```python
from build123d import *

# Parameters (mm, degrees)
SKETCH1_R           = 7
BOSS_EXTRUDE1_DEPTH = 2
SKETCH2_R           = 5.95
BOSS_EXTRUDE2_DEPTH = 7
SKETCH3_W           = 3.8
SKETCH3_H           = 3.8
CUT_EXTRUDE1_DEPTH  = 1.8
CHAMFER1_SIZE       = 1


with BuildPart() as part:
    # Sketch1 → Boss-Extrude1 (new body)
    with BuildSketch(Plane(origin=(0, 0, 0), x_dir=(1, 0, 0), z_dir=(0, 1, 0))):
        with Locations(Location((0, 0, 0), (0, 0, 270))):
            Circle(SKETCH1_R)
    extrude(amount=BOSS_EXTRUDE1_DEPTH)

    # Sketch2 → Boss-Extrude2 (add)
    with BuildSketch(Plane(origin=(0, 2, 0), x_dir=(1, 0, 0), z_dir=(0, 1, 0))):
        with Locations(Location((0, 0, 0), (0, 0, 270))):
            Circle(SKETCH2_R)
    extrude(amount=BOSS_EXTRUDE2_DEPTH)

    # Sketch3 → Cut-Extrude1 (cut)
    with BuildSketch(Plane.XZ):
        with BuildLine():
            ThreePointArc((-1.9, 1.9), (-2.687005769, 0), (-1.9, -1.9))
            Line((-1.9, -1.9), (-1.9, 1.9))
        make_face()
        Rectangle(SKETCH3_W, SKETCH3_H)
        with BuildLine():
            ThreePointArc((1.9, 1.9), (0, 2.687005769), (-1.9, 1.9))
            Line((-1.9, 1.9), (1.9, 1.9))
        make_face()
        with BuildLine():
            Line((1.9, 1.9), (1.9, -1.9))
            ThreePointArc((1.9, -1.9), (2.482469633, -1.02827259), (2.687005769, 0))
            ThreePointArc((2.687005769, 0), (2.482469633, 1.02827259), (1.9, 1.9))
        make_face()
        with BuildLine():
            Line((1.9, -1.9), (-1.9, -1.9))
            ThreePointArc((-1.9, -1.9), (0, -2.687005769), (1.9, -1.9))
        make_face()
    extrude(amount=-CUT_EXTRUDE1_DEPTH, mode=Mode.SUBTRACT)

    # Chamfer1
    chamfer1_edges = [part.edges().sort_by_distance(p)[0] for p in [
        (0, 9, -5.95),
    ]]
    chamfer(chamfer1_edges, length=CHAMFER1_SIZE)


solid = part.part
```
CAD build for the part. Positions are in the model's coordinates, mm. Round coordinates to 2 decimals unless told otherwise and drop trailing zeros. Order: outer loops, then holes, each group sorted by start corner. A loop starts at its lowest first (then second) coordinate and runs counter-clockwise, first axis right, second up. Notation, with made-up numbers: (-38, 52.25) -> (17, 52.25) arc R16 ccw to (17, 75.25) -> close; hole circle Ø7 at (18, -19.5). An arc over 180 degrees is marked (long way). Write item = value, one per line.
(1) Pull direction X, two halves, no side cores. Call faces 1 (the flat face through (0, 1.8, 0)), 2 (the flat face through (-6, 2, -2)), 3 (the cylindrical face through (1.787, 4.958, 5.675)): +X half, -X half, draft (parallel to the pull), parting line (faces both ways), or undercut.
Answers follow:
face_1 = undercut
face_2 = draft
face_3 = parting line
(2) Flat gauge pins, fed straight in: P1, Ø3, axis at y = 4.5, z = -0.5, coming from the +X side; P2, Ø1, axis at x = 0, y = 5, coming from the +Z side; P3, Ø1.5, axis at y = 7.5, z = -5, coming from the -X side. Where does each tip first touch, or does it go through?
Answers follow:
P1 = 5.95
P2 = 5.95
P3 = -4.16
(3) Cut at B-B (y = 1). Write the cut outline in (x, z).
Answers follow:
outline = circle Ø14 at (0, 0); hole circle Ø5.37 at (0, 0)
(4) Cut at D-D (y = 8.25). Write the cut outline in (x, z), plus the area to 3 significant figures.
Answers follow:
outline = circle Ø11.4 at (0, 0)
area = 102 mm²
(5) Cut at C-C (y = 3.25). Write the cut outline in (x, z), plus the area to 3 significant figures.
Answers follow:
outline = circle Ø11.9 at (0, 0)
area = 111 mm²
(6) Cut at A-A (x = 0). Write the cut outline in (y, z).
Answers follow:
outline = (0, -7) -> (2, -7) -> (2, -5.95) -> (8, -5.95) -> (9, -4.95) -> (9, 4.95) -> (8, 5.95) -> (2, 5.95) -> (2, 7) -> (0, 7) -> (0, 2.69) -> (1.8, 2.69) -> (1.8, -2.69) -> (0, -2.69) -> close
(7) Drill centre lines: L1, parallel to X at y = 1.75, z = 0.5; L2, parallel to Y at x = -6, z = -2.25. Where is each one in solid material? Low to high.
Answers follow:
L1 = -6.98 to -2.64, 2.64 to 6.98
L2 = 0 to 2
